from build123d import *

# Parameters (mm, degrees)
BOSS_EXTRUDE1_DEPTH = 64.45
BOSS_EXTRUDE2_DEPTH = 11.14
BOSS_EXTRUDE3_DEPTH = 2.46
BOSS_EXTRUDE4_DEPTH = 25


with BuildPart() as part:
    # Sketch1 → Boss-Extrude1 (new, symmetric)
    with BuildSketch(Plane.XY):
        with BuildLine():
            Line((-11.1, 11.315), (11.1, 11.315))
            ThreePointArc((11.1, 11.315), (22.415, 0), (11.1, -11.315))
            Line((11.1, -11.315), (-11.1, -11.315))
            ThreePointArc((-11.1, -11.315), (-22.415, 0), (-11.1, 11.315))
        make_face()
    extrude(amount=BOSS_EXTRUDE1_DEPTH, both=True)

    # Sketch2 → Boss-Extrude2 (add)
    with BuildSketch(Plane.XY.offset(64.45)):
        with BuildLine():
            Line((-11.1, -11.95), (11.1, -11.95))
            ThreePointArc((11.1, -11.95), (23.05, 0), (11.1, 11.95))
            Line((11.1, 11.95), (-11.1, 11.95))
            ThreePointArc((-11.1, 11.95), (-23.05, 0), (-11.1, -11.95))
        make_face()
    boss_extrude2 = extrude(amount=-BOSS_EXTRUDE2_DEPTH)

    # Mirror1: Boss-Extrude2 across plane
    add(boss_extrude2.mirror(Plane.XY))

    # Sketch3 → Boss-Extrude3 (add)
    with BuildSketch(Plane.XY.offset(64.45)):
        with BuildLine():
            Line((-11.25, 6.45), (11.25, 6.45))
            ThreePointArc((11.25, 6.45), (17.7, 0), (11.25, -6.45))
            Line((11.25, -6.45), (-11.25, -6.45))
            ThreePointArc((-11.25, -6.45), (-17.7, 0), (-11.25, 6.45))
        make_face()
    extrude(amount=BOSS_EXTRUDE3_DEPTH)

    # Sketch4 → Boss-Extrude4 (add)
    with BuildSketch(Plane.XY.offset(66.91)):
        with BuildLine():
            Line((-2.875, 3.125), (2.875, 3.125))
            ThreePointArc((2.875, 3.125), (6, 0), (2.875, -3.125))
            Line((2.875, -3.125), (-2.875, -3.125))
            ThreePointArc((-2.875, -3.125), (-6, 0), (-2.875, 3.125))
        make_face()
    extrude(amount=BOSS_EXTRUDE4_DEPTH)


solid = part.part
CAD build for the part. Positions are in the model's coordinates, mm. A direction names the side the tool comes from. Give positions to 0.01 mm unless a question says otherwise; leave off trailing zeros. Order: outer loops, then holes, each group sorted by start corner. A loop starts at its lowest first (then second) coordinate and runs counter-clockwise, first axis right, second up. Notation, with made-up numbers: (68, 43.25) - (122, 43.25) arc R22 cw to (122, 65.25) - close; hole circle Ø6 at (3, 80). An arc over 180 degrees is marked (long way). Answer in a Markdown table with one row per item.
1. Probe probe 1 along X at (y, z) = (-0.25, 51); probe 2 along Z at (x, y) = (-8, -5.5); probe 3 along Y at (x, z) = (-11, 39) (3 decimals). List the from-to ranges inside material, lowest first. Write a range as [from, to].
Data:
| item | result |
|---|---|
| probe 1 | x = [-22.41, 22.41] |
| probe 2 | z = [-64.45, 66.91] |
| probe 3 | y = [-11.315, 11.315] |
2. Saw through at A-A, the plane y = 0. Give the cut face in (x, z) (3 decimals).
Data:
| item | result |
|---|---|
| outline | (-23.05, -64.45) - (23.05, -64.45) - (23.05, -53.31) - (22.415, -53.31) - (22.415, 53.31) - (23.05, 53.31) - (23.05, 64.45) - (17.7, 64.45) - (17.7, 66.91) - (6, 66.91) - (6, 91.91) - (-6, 91.91) - (-6, 66.91) - (-17.7, 66.91) - (-17.7, 64.45) - (-23.05, 64.45) - (-23.05, 53.31) - (-22.415, 53.31) - (-22.415, -53.31) - (-23.05, -53.31) - close |
3. Tool access for faces 4 (the flat face through (0, -3.125, 79)), 5 (the flat face through (0, -11.315, 1)), 6 (the cylindrical face through (-6, 0, 79)): list every direction of +Z, -Z, +X, -X, +Y, -Y with a clear straight run to the whole face (end or side of a thin tool).
Data:
| item | result |
|---|---|
| face 4 | +Z, +X, -X, -Y |
| face 5 | +X, -X, -Y |
| face 6 | +Z, -X |
4. Saw through at C-C, the plane z = 1. Give the cut face in (x, y) (3 decimals).
Data:
| item | result |
|---|---|
| outline | (-11.1, -11.315) - (11.1, -11.315) arc R11.315 ccw to (11.1, 11.315) - (-11.1, 11.315) arc R11.315 ccw to start |
5. Saw through at B-B, the plane x = 16. Give the cut face in (y, z).
Data:
| item | result |
|---|---|
| outline | (-10.9, -64.45) - (10.9, -64.45) - (10.9, -53.31) - (10.2, -53.31) - (10.2, 53.31) - (10.9, 53.31) - (10.9, 64.45) - (4.36, 64.45) - (4.36, 66.91) - (-4.36, 66.91) - (-4.36, 64.45) - (-10.9, 64.45) - (-10.9, 53.31) - (-10.2, 53.31) - (-10.2, -53.31) - (-10.9, -53.31) - close |
6. Flat gauge pins, fed straight in: pin 1 (8 mm diameter, centred on x = 14, z = -7, fed in from -Y) (3 decimals); pin 2 (12 mm diameter, centred on x = 11.5, z = -48, fed in from +Y); pin 3 (6.5 mm diameter, centred on x = 0, z = 75, fed in from -Y) (3 decimals); pin 4 (4 mm diameter, centred on y = 6, z = -17, fed in from +X). Where does each tip first touch, or does it go through?
Data:
| item | result |
|---|---|
| pin 1 | stops at y = -11.315 |
| pin 2 | stops at y = 11.95 |
| pin 3 | stops at y = -3.125 |
| pin 4 | stops at x = 21.68 |
7. Pull direction Z, two halves, no side cores. Call faces 1 (the cylindrical face through (-22.412, -0.249, 0.746)), 2 (the flat face through (0, 8, 64.45)), 3 (the cylindrical face through (-23.047, 0.263, 58.958)): pulls with the +Z half, pulls with the -Z half, needs draft (parallel to the pull), parting line crosses it, or undercut.
Data:
| item | result |
|---|---|
| face 1 | undercut |
| face 2 | pulls with the +Z half |
| face 3 | needs draft |
